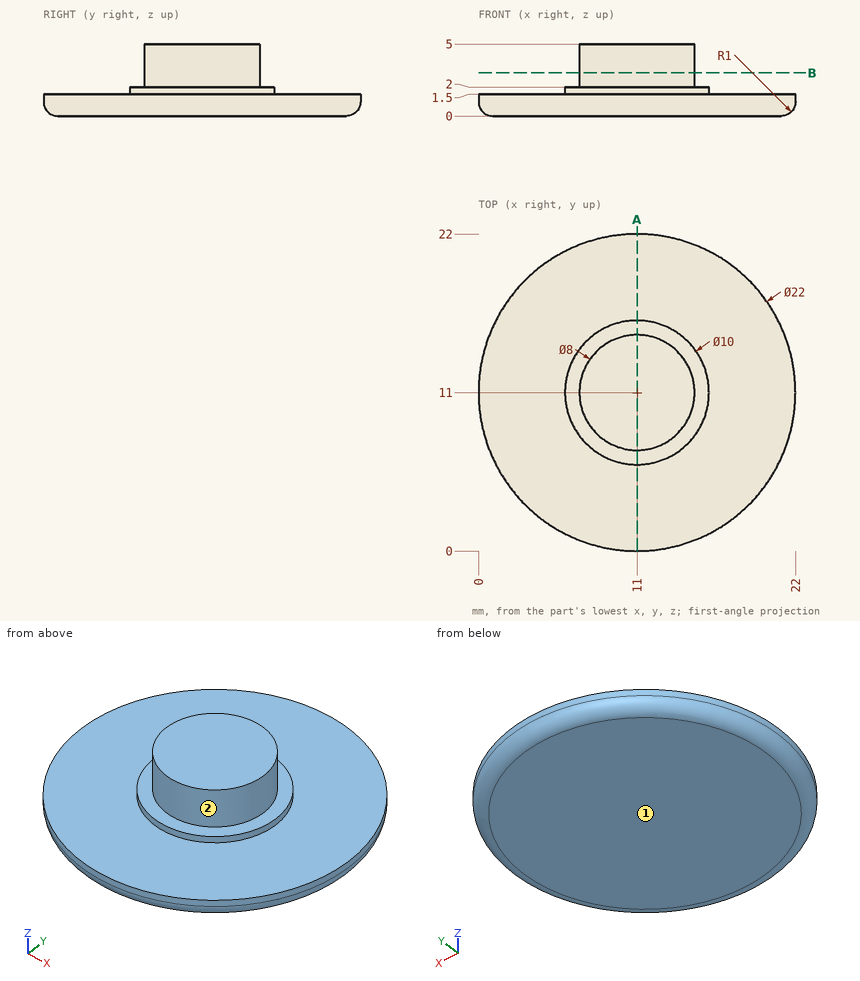
Could you check a few things on this drawing? It's one solid part, dimensions in mm from its lowest x, y, z. A direction names the side the tool comes from. Round coordinates to 2 decimals unless told otherwise and drop trailing zeros. Order: outer loops, then holes, each group sorted by start corner. A loop starts at its lowest first (then second) coordinate and runs counter-clockwise, first axis right, second up. Notation, with made-up numbers: M -10,77 L 30,77 A23 cw 30,110 Z; hole C -10.75,71 d6. An arc over 180 degrees is marked long. Use a Markdown table: item, result.
1) I'm going to push flat-ended pins straight in: P1, Ø1, axis at x = 8.5, z = 4, coming from the -Y side; P2, Ø12, axis at x = 14.5, y = 5.5, coming from the +Z side. Where does each tip first touch, or does it pass through?
Geometry says:
| item | result |
|---|---|
| P1 | stops at y = 7.54 |
| P2 | stops at z = 5 |
2) Imagine slicing it at B-B (z = 3). List the corners of the cut face in (x, y) for me, then the cut area to 3 significant figures.
Geometry says:
| item | result |
|---|---|
| outline | C 11,11 d8 |
| area | 50.3 mm² |
3) If I drill on line 1 along Z through (x, y) = (16.5, 17.5); line 2 along Z through (x, y) = (9, 7.5); line 3 along Y through (x, z) = (13.25, 2.05), over which ranges is the centre line in solid material (lowest first)?
Geometry says:
| item | result |
|---|---|
| line 1 | z = 0 to 1.5 |
| line 2 | z = 0 to 2 |
| line 3 | y = 7.69 to 14.31 |
4) On a 3-axis mill with a long thin cutter (end or side, diameter ignored), from which of +Z, -Z, +X, -X, +Y, -Y can I reach the whole of each face in a straight line? I mean the marked faces 1 and 2. Say none if no direction works.
Geometry says:
| item | result |
|---|---|
| face 1 | -Z, +X, -X, +Y, -Y |
| face 2 | +Z |
5) Imagine slicing it at A-A (x = 11). List the corners of the cut face in (y, z) for me, then the cut area to 3 significant figures.
Geometry says:
| item | result |
|---|---|
| outline | M 0,1 A1 ccw 1,0 L 21,0 A1 ccw 22,1 L 22,1.5 L 16,1.5 L 16,2 L 15,2 L 15,5 L 7,5 L 7,2 L 6,2 L 6,1.5 L 0,1.5 Z |
| area | 61.6 mm² |
